Autodesk Fusion 360 part; units mm, degrees
sketch "Sketch1" plane through (0, 0, 0) normal (0, 1, 0) x (1, 0, 0)
  line L0 (0, 0) -> (5, 0)
  line L1 (5, 0) -> (5, -10.5)
  line L2 (5, -10.5) -> (0, -10.5)
  line L3 (0, -10.5) -> (0, 0)
  line L4 (5, -10.5) -> (5, -12)
  line L5 (5, -12) -> (3.5, -12)
  circle A0 centre (0, -10.5) radius 0.5
  line L6 (3.5, -12) -> (0.5, -10.5)
  line L7 (0, 0) -> (0, -5.6)
  line L8 (0, -5.6) -> (2.5, -5.6)
  line L9 (2.5, -5.6) -> (5, -10.5)
  point P0 (0, -10)
  dimension "d1" = 5
  dimension "d2" = 10.5
  dimension "d3" = 1
  dimension "d7" = 1.5
  dimension "d8" = 1.5
  dimension "d9" = 5.6
  dimension "d10" = 2.5
revolve "Revolve1" add sketch "Sketch1" angle 360 about axis through (1.75, 0, 0) along (1, 0, 0) contours L2 L3 A0 L8 L9 | L2 L4 L5 L6
mirror "Mirror1" about plane through (0, 0, 0) normal (1, 0, 0) of bodies 1 merged
sketch "Sketch2" plane through (0, 0, 0) normal (0, 1, 0) x (1, 0, 0)
  line L0 (0, 0) -> (5, 0)
  line L1 (5, 0) -> (5, -10.5)
  line L2 (2.5, 0) -> (2.5, -5.6)
  line L3 (5, -10.5) -> (2.5, -5.6)
  line L4 (3.5, 0) -> (3.5, -7.56)
  line L5 (2.5, -4.6) -> (3.5, -4.6)
  dimension "d11" = 10.5
  dimension "d12" = 5.6
  dimension "d13" = 1
  dimension "d14" = 1
revolve "Revolve2" add sketch "Sketch2" angle 360 about axis through (0, 0, 0) along (1, 0, 0) contours L2 L3 L4 L5
Geometry check sheet. Reference: the model listing, model coordinates, mm. A direction names the side the tool comes from. Round coordinates to 2 decimals unless told otherwise and drop trailing zeros. Loops run counter-clockwise (first coordinate to the right, second up) from the corner with the lowest first, then second, coordinate; pieces in that order, holes last. Notation, with made-up numbers: (0.25, 68) - (20.25, 68) arc R31 ccw to (20.25, 101) - close; hole circle Ø6 at (-11, 52.5). An arc over 180 degrees is marked (long way). Use a Markdown table: item, result.
Q1. Cross-section at A-A on y = 0. Record the cut outline in (x, z), plus the area to 3 significant figures.
Solutions:
| item | result |
|---|---|
| outline | (-5, -12) - (-3.5, -12) - (-0.5, -10.5) arc R0.5 cw to (0.5, -10.5) - (3.5, -12) - (5, -12) - (5, -10.5) - (3.5, -7.56) - (3.5, -4.6) - (2.5, -4.6) - (2.5, -5.6) - (-2.5, -5.6) - (-5, -10.5) - close; (-5, 10.5) - (-2.5, 5.6) - (2.5, 5.6) - (2.5, 4.6) - (3.5, 4.6) - (3.5, 7.56) - (5, 10.5) - (5, 12) - (3.5, 12) - (0.5, 10.5) arc R0.5 cw to (-0.5, 10.5) - (-3.5, 12) - (-5, 12) - close |
| area | 94.7 mm2 |
Q2. Draft check along Z on faces 1 (the cylindrical face through (-4.24, -0.53, -11.99)), 2 (the flat face through (2.5, -5, 0)), 3 (the flat face through (5, 11, 0)). Enter one of: released by +Z, released by -Z, zero draft, split by the parting line, or undercut.
Solutions:
| item | result |
|---|---|
| face 1 | split by the parting line |
| face 2 | undercut |
| face 3 | zero draft |
Q3. Go/stop test with flat-tipped pins: P1, Ø5, axis at x = -3.5, z = -8.5, coming from the +Y side; P2, Ø7.5, axis at y = -1.5, z = -0.5, coming from the +X side; P3, Ø6, axis at x = -2.5, z = -8, coming from the -Y side; P4, Ø8.5, axis at y = 0, z = 0, coming from the -X side. Record where each tip stops, or that it passes through.
Solutions:
| item | result |
|---|---|
| P1 | stops at y = 10.39 |
| P2 | stops at x = 3.5 |
| P3 | stops at y = -10.83 |
| P4 | passes through |
Q4. Access from +Z, -Z, +X, -X, +Y, -Y to the whole of each face (thin tool, end or side, straight path). Record for faces 4 (the flat face through (3.5, 5, 0)), 5 (the cylindrical face through (0.035, -0.246, -5.595)), 6 (the conical face through (-0.688, 10.504, -1.379)), 7 (the flat face through (-5, 11, 0)).
Solutions:
| item | result |
|---|---|
| face 4 | +X |
| face 5 | -X |
| face 6 | none |
| face 7 | +Z, -Z, -X, +Y, -Y |
Q5. Material ranges on line 1 (Z direction, x = 1.25, y = -0.25); line 2 (X direction, y = -5, z = -2.25); line 3 (Z direction, x = 3.05, y = 0) (3 decimals), recorded low to high.
Solutions:
| item | result |
|---|---|
| line 1 | z = -10.87 to -5.59, 5.59 to 10.87 |
| line 2 | x = 2.5 to 3.5 |
| line 3 | z = -11.775 to -4.6, 4.6 to 11.775 |
Q6. Cross-section at C-C on x = -4. Record the cut outline in (y, z), plus the area to 3 significant figures.
Solutions:
| item | result |
|---|---|
| outline | circle Ø24 at (0, 0); hole circle Ø17.08 at (0, 0) |
| area | 223 mm2 |
